Autodesk Inventor part; units mm, degrees
ref_plane "YZ Plane" through (0, 0, 0) normal (1, 0, 0) x (0, 1, 0)
ref_plane "XZ Plane" through (0, 0, 0) normal (0, 1, 0) x (-1, 0, 0)
ref_plane "XY Plane" through (0, 0, 0) normal (0, 0, 1) x (1, 0, 0)
sketch "Sketch1" plane through (0, 0, 0) normal (0, 0, 1) x (1, 0, 0)
  arc A0 (6.75, 0) -> (-6.75, 0) centre (0, 0) ccw
  arc A1 (9.75, 0) -> (-9.75, 0) centre (0, 0) ccw
  line L0 (-6.75, 0) -> (-9.75, 0)
  line L1 (6.75, 0) -> (9.75, 0)
  dimension "d0" = 13.5
  dimension "d1" = 3
extrude "Extrusion1" add sketch "Sketch1" along normal blind 10
sketch "Sketch2" plane through (-9.75, 0, 0) normal (0, -1, 0) x (1, 0, 0)
  line L0 (3, 0) -> (3, 10)
  line L1 (3, 0) -> (-7.1864, 0)
  line L2 (-7.1864, 0) -> (-7.1864, 10)
  line L3 (-7.1864, 10) -> (3, 10)
  line L4 (3, 10) -> (3, 0)
  point P0 (9.75, 0)
  dimension "d14" = 10
extrude "Extrusion2" add sketch "Sketch2" along normal blind 3
ref_plane "Work Plane1" through (0, -3, 10) normal (1, 0, 0) x (0, 0, -1)
mirror "Mirror1" about plane through (0, -3, 10) normal (1, 0, 0) of "Extrusion2"
sketch "Sketch3" plane through (-9.75, 0, 0) normal (0, 1, 0) x (1, 0, 0)
  line L0 (0, -10) -> (19.5, -10)
  line L1 (-7.1864, 0) -> (3, 0)
  line L2 (9.75, 0) -> (9.75, -10)
  line L3 (3, -10) -> (16.5, -10)
  point P0 (-3.5932, -5)
  point P1 (23.0932, -5)
  dimension "d15" = 5
hole "Hole1" at (-13.3432, 0, 5) at (13.3432, 0, 5) direction (0, -1, 0) diameter 4.5 end through all
fillet "Fillet1" radius 2 4 edges at (16.9364, -1.5, 10) (16.9364, -1.5, 0) (-16.9364, -1.5, 10) (-16.9364, -1.5, 0)
properties part number "Eletronica - Trava cabo"
The listing builds one solid part. Answer for the finished solid, in the listing's coordinates (mm). A direction names the side the tool comes from. Coordinates: 2 decimals unless noted, no trailing zeros. Write each loop counter-clockwise with the first axis right and the second up, starting at its lowest first coordinate (ties: lowest second). Pieces come first, ordered by that corner, then holes. Notation, with made-up numbers: M 69,29 L 90,29 A26 ccw 90,59 Z; hole C 40.25,85 d10. An arc over 180 degrees is marked long. Write each question's results on one line, items separated by ' | '.
Item 1: For a pull along Z with two mould halves and no side action, classify faces 1 (the face through (11.446, -1.521, 6.21)), 2 (the face through (0, 7, 10)), 3 (the face through (-12.6, 0, 7.3)) as released by +Z, released by -Z, zero draft, split by the parting line, or undercut.
Answer below:
face 1: undercut | face 2: released by +Z | face 3: zero draft
Item 2: The part is cut by section C-C on y = -1. Determine the outline of the cut face in (x, z), and give its area (3 significant figures).
Answer below:
outline: M -16.94,2 A2 ccw -14.94,0 L -6.75,0 L -6.75,10 L -14.94,10 A2 ccw -16.94,8 Z; M 6.75,0 L 14.94,0 A2 ccw 16.94,2 L 16.94,8 A2 ccw 14.94,10 L 6.75,10 Z; hole C -13.34,5 d4.5; hole C 13.34,5 d4.5 | area: 168 mm2
Item 3: Which of the six approach directions +Z, -Z, +X, -X, +Y, -Y give full straight-line access (tool end or side, diameter ignored) to faces 4 (the face through (-6.75, -1, 5)), 5 (the face through (16.335, -1.521, 0.57)), 6 (the face through (10.9, 0, 5.1))?
Answer below:
face 4: +Z, -Z, -Y | face 5: -Z, +X, +Y, -Y | face 6: +Z, -Z, +X, +Y
Item 4: Given P1, Ø4, axis at x = 3.5, z = 4, coming from the -Y side; P2, Ø5, axis at x = -13.34, z = 5, coming from the +Y side; P3, Ø1.5, axis at x = -1.5, z = 2, coming from the -Y side, each flat-ended and moving along its own axis, determine where each tip first touches the part or whether it passes through.
Answer below:
P1: y = 3.91 | P2: y = 0 | P3: y = 6.36
Item 5: The part is cut by section A-A on z = 5. Determine the outline of the cut face in (x, y).
Answer below:
outline: M -16.94,-3 L -15.59,-3 L -15.59,0 L -16.94,0 Z; M -11.09,-3 L -6.75,-3 L -6.75,0 A6.75 cw 6.75,0 L 6.75,-3 L 11.09,-3 L 11.09,0 L 9.75,0 A9.75 ccw -9.75,0 L -11.09,0 Z; M 15.59,-3 L 16.94,-3 L 16.94,0 L 15.59,0 Z
Item 6: The part is cut by section D-D on x = -13. Determine the outline of the cut face in (y, z), and give its area (3 significant figures).
Answer below:
outline: M -3,0 L 0,0 L 0,2.78 L -3,2.78 Z; M -3,7.22 L 0,7.22 L 0,10 L -3,10 Z | area: 16.7 mm2
Item 7: Consider probe 1 along X at (y, z) = (-0.95, 5); probe 2 along X at (y, z) = (4, 4.25); probe 3 along X at (y, z) = (-2.5, 3). Determine where each line is inside the solid, lowest interval first. Write a range as [from, to].
Answer below:
probe 1: [-16.94, -15.59], [-11.09, -6.75], [6.75, 11.09], [15.59, 16.94] | probe 2: [-8.89, -5.44], [5.44, 8.89] | probe 3: [-16.94, -14.37], [-12.31, -6.75], [6.75, 12.31], [14.37, 16.94]
Item 8: The part is cut by section B-B on y = 1.25. Determine the outline of the cut face in (x, z), and give its area (3 significant figures).
Answer below:
outline: M -9.67,0 L -6.63,0 L -6.63,10 L -9.67,10 Z; M 6.63,0 L 9.67,0 L 9.67,10 L 6.63,10 Z | area: 60.7 mm2
